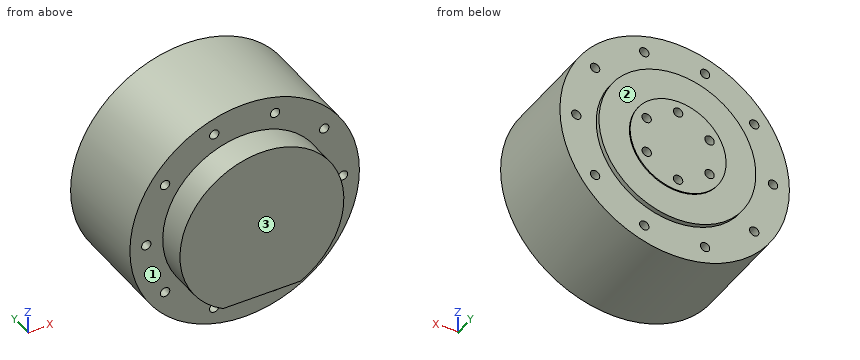
```python
from build123d import *

# Parameters (mm, degrees)
SKETCH_1_R               = 49
EXTRUDE_1_DEPTH          = 43
SKETCH_2_R               = 33.5
EXTRUDE_2_DEPTH          = 2
EXTRUDE_3_DEPTH          = 12.5
SKETCH_4_R               = 20.5
EXTRUDE_4_DEPTH          = 0.5
SKETCH_5_R               = 2
CUT_EXTRUDE_1_DEPTH      = 5
PATTERN_CIRCULAR_1_COUNT = 6
SKETCH_6_R               = 2
CUT_EXTRUDE_2_DEPTH      = 5
PATTERN_CIRCULAR_2_COUNT = 10
CUT_EXTRUDE_START        = -5
SKETCH_7_R               = 2
CUT_EXTRUDE_3_DEPTH      = 5
PATTERN_CIRCULAR_3_COUNT = 10


with BuildPart() as part:
    # 草圖1 → 填料-伸長1 (new body)
    with BuildSketch(Plane(origin=(0, 0, 0), x_dir=(1, 0, 0), z_dir=(0, 1, 0))):
        with Locations(Location((0, 0, 0), (0, 0, 270))):
            Circle(SKETCH_1_R)
    extrude(amount=EXTRUDE_1_DEPTH)

    # 草圖2 → 填料-伸長2 (add)
    with BuildSketch(Plane(origin=(0, 43, 0), x_dir=(1, 0, 0), z_dir=(0, 1, 0))):
        with Locations(Location((0, 0, 0), (0, 0, 270))):
            Circle(SKETCH_2_R)
    extrude(amount=EXTRUDE_2_DEPTH)

    # 草圖3 → 填料-伸長3 (add)
    with BuildSketch(Plane.XZ):
        with BuildLine():
            Line((-16.624078922, -30.8), (16.624078922, -30.8))
            ThreePointArc((16.624078922, -30.8), (0, 35), (-16.624078922, -30.8))
        make_face()
    extrude(amount=EXTRUDE_3_DEPTH)

    # 草圖4 → 填料-伸長4 (add)
    with BuildSketch(Plane(origin=(0, 45, 0), x_dir=(1, 0, 0), z_dir=(0, 1, 0))):
        with Locations(Location((0, 0, 0), (0, 0, 270))):
            Circle(SKETCH_4_R)
    extrude(amount=EXTRUDE_4_DEPTH)

    # 草圖5 → 除料-伸長1 (cut)
    with BuildSketch(Plane(origin=(0, 45.5, 0), x_dir=(1, 0, 0), z_dir=(0, 1, 0))):
        with Locations(Location((0, 15.5, 0), (0, 0, 270))):
            Circle(SKETCH_5_R)
    cut_extrude_1 = extrude(amount=-CUT_EXTRUDE_1_DEPTH, mode=Mode.SUBTRACT)

    # 環狀複製排列1: 除料-伸長1 ×6 about axis
    pattern_circular_1_axis = Axis((0, 0, 0), (0, 1, 0))
    for i in range(1, PATTERN_CIRCULAR_1_COUNT):
        add(cut_extrude_1.rotate(pattern_circular_1_axis, i * 360 / PATTERN_CIRCULAR_1_COUNT), mode=Mode.SUBTRACT)

    # 草圖6 → 除料-伸長2 (cut)
    with BuildSketch(Plane(origin=(0, 43, 0), x_dir=(1, 0, 0), z_dir=(0, 1, 0))):
        with Locations(Location((-42, 0, 0), (0, 0, 270))):
            Circle(SKETCH_6_R)
    cut_extrude_2 = extrude(amount=-CUT_EXTRUDE_2_DEPTH, mode=Mode.SUBTRACT)

    # 環狀複製排列2: 除料-伸長2 ×10 about axis
    pattern_circular_2_axis = Axis((0, 0, 0), (0, 1, 0))
    for i in range(1, PATTERN_CIRCULAR_2_COUNT):
        add(cut_extrude_2.rotate(pattern_circular_2_axis, i * 360 / PATTERN_CIRCULAR_2_COUNT), mode=Mode.SUBTRACT)

    # 草圖7 → 除料-伸長3 (cut)
    with BuildSketch(Plane.XZ.offset(CUT_EXTRUDE_START)):
        with Locations(Location((42, 0, 0), (0, 0, 270))):
            Circle(SKETCH_7_R)
    cut_extrude_3 = extrude(amount=CUT_EXTRUDE_3_DEPTH, mode=Mode.SUBTRACT)

    # 環狀複製排列3: 除料-伸長3 ×10 about axis
    pattern_circular_3_axis = Axis((0, 0, 0), (0, 1, 0))
    for i in range(1, PATTERN_CIRCULAR_3_COUNT):
        add(cut_extrude_3.rotate(pattern_circular_3_axis, i * 360 / PATTERN_CIRCULAR_3_COUNT), mode=Mode.SUBTRACT)


solid = part.part
```
Here's how the part is built. I have some questions about the finished solid (model axes, mm). Face numbers are marked on the shaded views. A direction names the side the tool comes from. Give positions to 0.01 mm unless a question says otherwise; leave off trailing zeros. Write each loop counter-clockwise with the first axis right and the second up, starting at its lowest first coordinate (ties: lowest second). Pieces come first, ordered by that corner, then holes. Notation, with made-up numbers: (53, 84.25) -> (69, 84.25) arc R24 ccw to (69, 99.25) -> close; hole circle Ø4 at (64, 69.5). An arc over 180 degrees is marked (long way). Use one line per item in the form item = value.
1) I'm going to push flat-ended pins straight in: pin 1 (3.5 mm diameter, centred on x = 12.98, z = 39.94, fed in from +Y); pin 2 (2 mm diameter, centred on x = 28, z = 6.5, fed in from +Y); pin 3 (3 mm diameter, centred on x = 7, y = -0.5, fed in from +Z). Where does each tip first touch, or does it pass through?
Verdict:
pin_1 = 38
pin_2 = 45
pin_3 = 48.68
2) On a 3-axis mill with a long thin cutter (end or side, diameter ignored), from which of +Z, -Z, +X, -X, +Y, -Y can I reach the whole of each face in a straight line? I mean the marked faces 1, 2 and 3. Say none if no direction works.
Verdict:
face_1 = -Y
face_2 = +Y
face_3 = +Z, -Z, +X, -X, -Y
3) If I drill on L1, parallel to X at y = 1, z = -23.5; L2, parallel to Y at x = -8, z = -36; L3, parallel to Y at x = -18, z = -12, over which ranges is the centre line in solid material (lowest first)? Write a range as [from, to].
Verdict:
L1 = [-43, -35.59], [-32.37, 32.37], [35.59, 43]
L2 = [0, 43]
L3 = [-12.5, 45]
4) Suppose I cut it at D-D (z = 30). Please give me the cut outline in (x, y), and give its area (3 significant figures).
Verdict:
outline = (-38.74, 0) -> (-18.03, 0) -> (-18.03, -12.5) -> (18.03, -12.5) -> (18.03, 0) -> (38.74, 0) -> (38.74, 43) -> (14.91, 43) -> (14.91, 45) -> (-14.91, 45) -> (-14.91, 43) -> (-38.74, 43) -> close
area = 3,840 mm2
5) Suppose I cut it at C-C (x = -42). Please give me the cut outline in (y, z).
Verdict:
outline = (0, -25.24) -> (43, -25.24) -> (43, -2) -> (38, -2) -> (38, 2) -> (43, 2) -> (43, 25.24) -> (0, 25.24) -> (0, 2) -> (5, 2) -> (5, -2) -> (0, -2) -> close
6) Suppose I cut it at B-B (y = 36). Please give me the cut outline in (x, z), and give its area (3 significant figures).
Verdict:
outline = circle Ø98 at (0, 0)
area = 7,540 mm2
